Job drawing, mm, ordinate dimensions from the low corner. One solid piece. A direction names the side the tool comes from. Coordinates: 2 decimals unless noted, no trailing zeros. Order: outer loops, then holes, each group sorted by start corner. A loop starts at its lowest first (then second) coordinate and runs counter-clockwise, first axis right, second up. Notation, with made-up numbers: (35.25, 54.25) - (92.25, 54.25) arc R14 cw to (92.25, 78.25) - close; hole circle Ø9 at (7, 87). An arc over 180 degrees is marked (long way). Return JSON: item names as keys, results as strings.
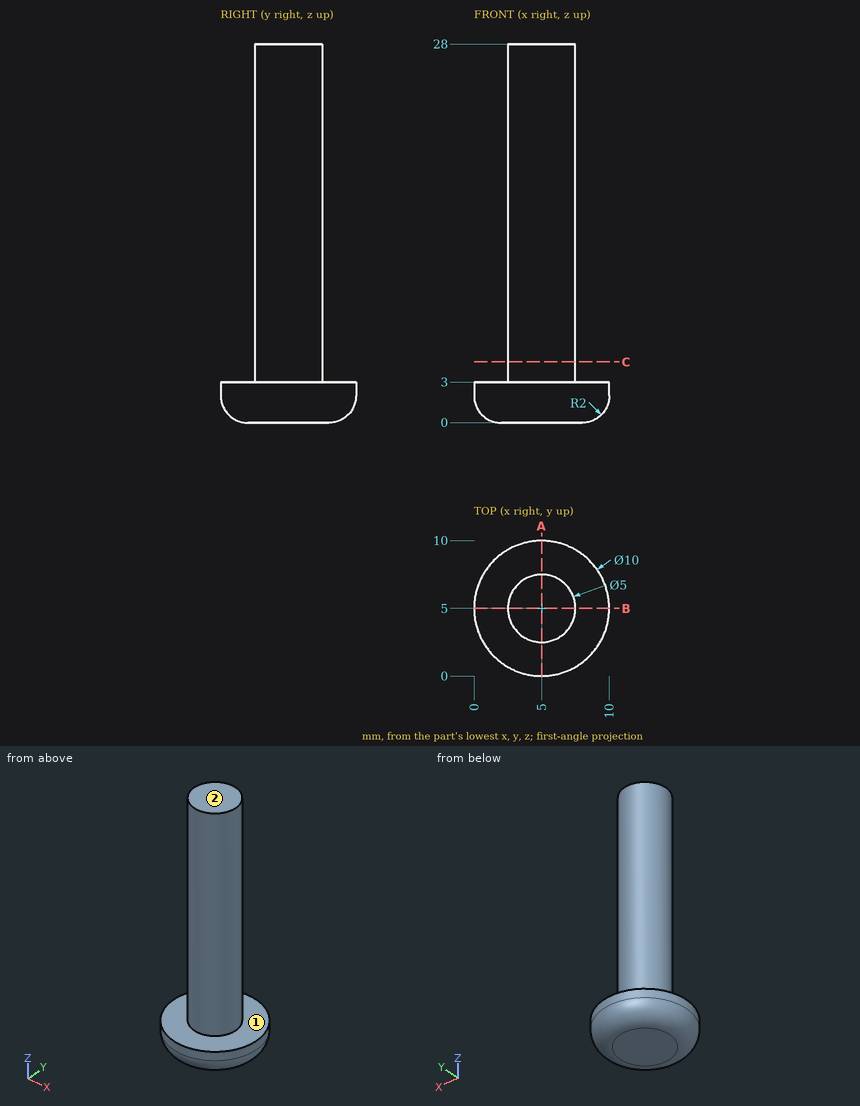
1. Drop flat-ended pins along their axis: pin 1 (4 mm diameter, centred on x = 2.5, z = 11.5, fed in from +Y); pin 2 (3 mm diameter, centred on x = 1.5, z = 5.5, fed in from -Y); pin 3 (3 mm diameter, centred on y = 6, z = 7, fed in from -X). Give the stop position or say it passes through.
Check values:
{"pin 1": "y = 7.45", "pin 2": "y = 3.5", "pin 3": "x = 2.5"}
2. Probe L1, parallel to Y at x = 5, z = 4.5; L2, parallel to Z at x = 7.5, y = 6.5; L3, parallel to Y at x = 3, z = 16.5. List the from-to ranges inside material, lowest first.
Check values:
{"L1": "2.5 to 7.5", "L2": "0 to 3", "L3": "3.5 to 6.5"}
3. Cut at C-C on z = 4.5. Give the cut face in (x, y), plus the area to 3 significant figures.
Check values:
{"outline": "circle Ø5 at (5, 5)", "area": "19.6 mm²"}
4. Tool access for the marked faces 1 and 2: list every direction of +Z, -Z, +X, -X, +Y, -Y with a clear straight run to the whole face (end or side of a thin tool).
Check values:
{"face 1": "+Z", "face 2": "+Z, +X, -X, +Y, -Y"}
5. Cut at A-A on x = 5. Give the cut face in (y, z).
Check values:
{"outline": "(0, 2) arc R2 ccw to (2, 0) - (8, 0) arc R2 ccw to (10, 2) - (10, 3) - (7.5, 3) - (7.5, 28) - (2.5, 28) - (2.5, 3) - (0, 3) - close"}
